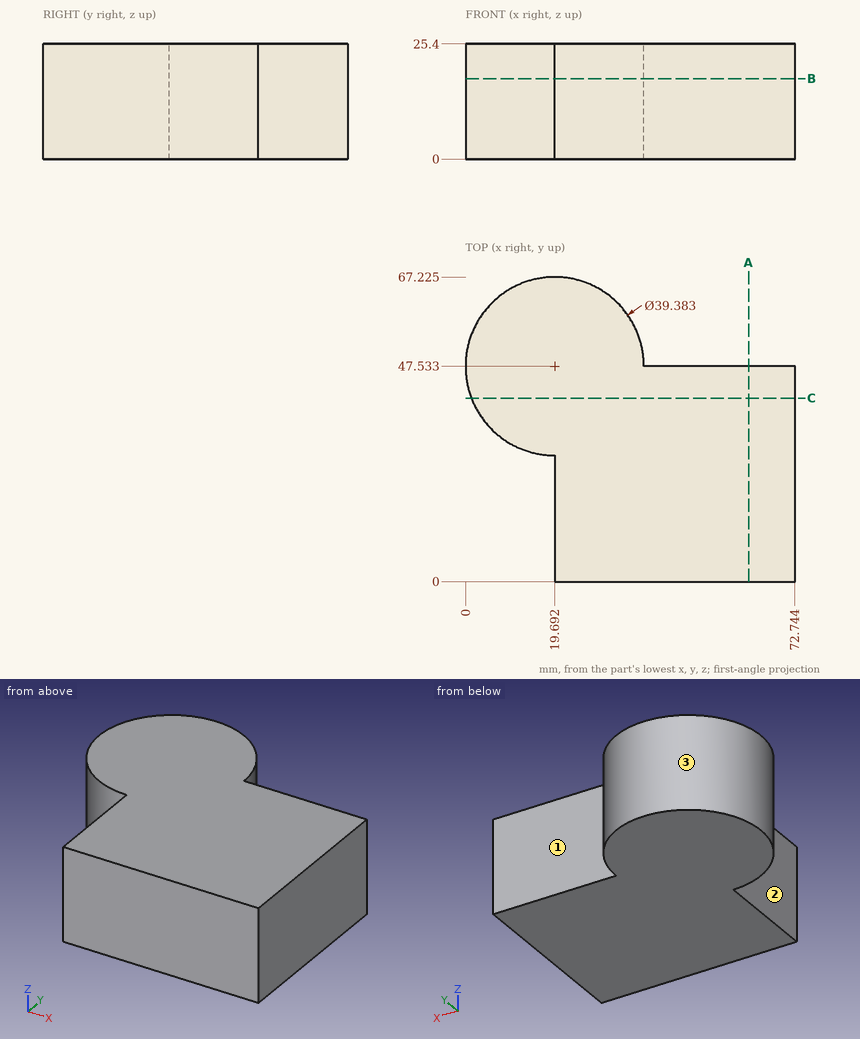
Geometry: see drawing. Coordinates: mm, zero at the bounding-box minimum. A direction names the side the tool comes from. Give positions to 0.01 mm unless a question says otherwise; leave off trailing zeros. Loops run counter-clockwise (first coordinate to the right, second up) from the corner with the lowest first, then second, coordinate; pieces in that order, holes last. Notation, with made-up numbers: (14.25, 40.5) -> (32.25, 40.5) arc R24 ccw to (32.25, 73.5) -> close; hole circle Ø10 at (-2, -24). An arc over 180 degrees is marked (long way). Answer as a JSON object with one key per item and string values. Group by question number.
Item 1: Reachability of the marked faces 1, 2 and 3 from +Z, -Z, +X, -X, +Y, -Y: full face, straight path, thin tool, end or side. Return the list, or none.
Item 2: Line query: probe 1 along X at (y, z) = (6.5, 16); probe 2 along Y at (x, z) = (25.5, 18.5); probe 3 along Y at (x, z) = (57, 11.5). Output: solid intervals per line, ascending.
Item 3: Cut plane C-C, the plane y = 40.5. Return the cut outline in (x, z).
Item 4: Cut plane B-B, the plane z = 17.75. Return the cut outline in (x, y), and give its area (3 significant figures).
Item 5: Pin query (flat end, axial travel): P1, Ø3, axis at x = 22, z = 5, coming from the +Y side; P2, Ø4, axis at x = 31.5, z = 16.5, coming from the +Y side; P3, Ø6, axis at x = 14, z = 3.5, coming from the -Y side. Return the tip coordinate at first contact, or that it passes through.
Item 6: Cut plane A-A, the plane x = 62.5. Return the cut outline in (y, z), and give its area (3 significant figures).
Checks:
{
 "1": {"face 1": "+Z, -Z, +X, +Y", "face 2": "+Z, -Z, -X, -Y", "face 3": "+Z, -Z"},
 "2": {"probe 1": "x = 19.69 to 72.74", "probe 2": "y = 0 to 66.35", "probe 3": "y = 0 to 47.53"},
 "3": {"outline": "(1.3, 0) -> (72.74, 0) -> (72.74, 25.4) -> (1.3, 25.4) -> close"},
 "4": {"outline": "(19.69, 0) -> (72.74, 0) -> (72.74, 47.53) -> (39.38, 47.53) arc R19.69 ccw (long way) to (19.69, 27.84) -> close", "area": "3,440 mm²"},
 "5": {"P1": "stops at y = 67.21", "P2": "stops at y = 64.61", "P3": "stops at y = 28.03"},
 "6": {"outline": "(0, 0) -> (47.53, 0) -> (47.53, 25.4) -> (0, 25.4) -> close", "area": "1,210 mm²"}
}
